Answer from the drawing. Dimensions are ordinates in mm from the lowest x, y and z of the part. Give positions to 0.01 mm unless a question says otherwise; leave off trailing zeros. Loops run counter-clockwise (first coordinate to the right, second up) from the corner with the lowest first, then second, coordinate; pieces in that order, holes last. Notation, with made-up numbers: (38, 86) - (94, 86) arc R24 ccw to (94, 98) - close; hole circle Ø7 at (85.25, 29). An arc over 180 degrees is marked (long way). Put each result on its own line as item: value. Start each with the question number.
1. Consider L1, parallel to X at y = 2.35, z = 25.4; L2, parallel to Z at x = 431.8, y = 1.75; L3, parallel to Z at x = 393.5, y = 20.25 (3 decimals). Determine where each line is inside the solid, lowest interval first. Write a range as from..to.
2. A cutting plane is placed at C-C, the plane z = 8.5. Determine the outline of the cut face in (x, y) (3 decimals).
3. A cutting plane is placed at A-A, the plane y = 17.25. Determine the outline of the cut face in (x, z) (3 decimals).
4. A cutting plane is placed at B-B, the plane x = 71. Determine the outline of the cut face in (y, z) (3 decimals), plus the area to 3 significant figures.
5. For a pull along Z with two mould halves and no side action, classify the marked faces 1, 2, 3 and 4 as released by +Z, released by -Z, zero draft, split by the parting line, or undercut.
6. Given pin 1 Ø8.5 at (x, z) = (25.4, 25.4) entering from +Y (3 decimals); pin 2 Ø2.5 at (y, z) = (14, 50) entering from +X; pin 3 Ø1.6 at (y, z) = (10, 49) entering from -X, each flat-ended and moving along its own axis, determine where each tip first touches the part or whether it passes through.
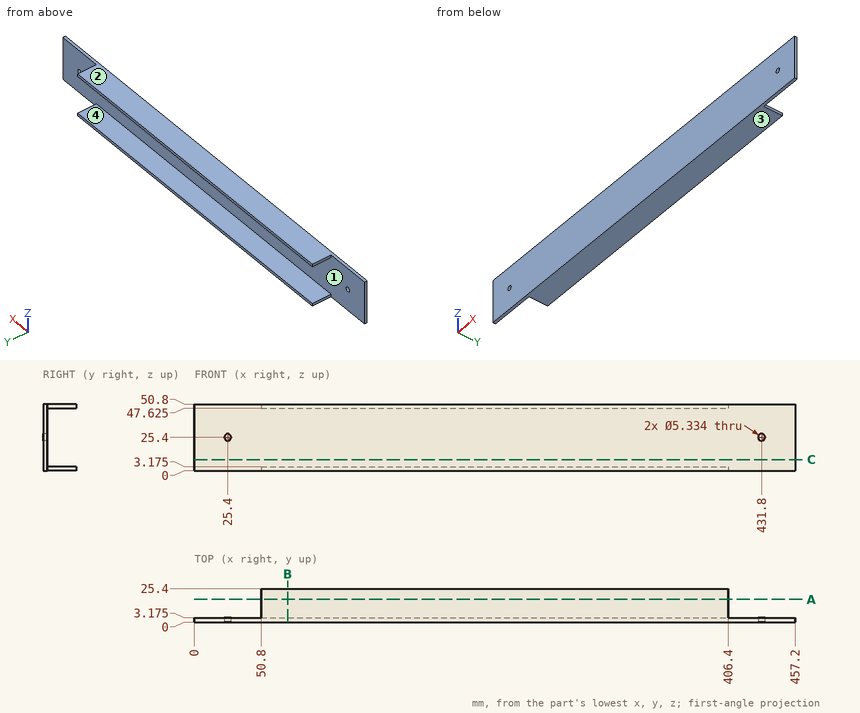
Return value:
1. L1: x = 0..22.73, 28.07..429.13, 434.47..457.2
1. L2: z = 0..22.73, 28.07..50.8
1. L3: z = 0..3.175, 47.625..50.8
2. outline: (0, 0) - (457.2, 0) - (457.2, 3.175) - (0, 3.175) - close
3. outline: (50.8, 0) - (406.4, 0) - (406.4, 3.175) - (50.8, 3.175) - close; (50.8, 47.625) - (406.4, 47.625) - (406.4, 50.8) - (50.8, 50.8) - close
4. outline: (0, 0) - (25.4, 0) - (25.4, 3.175) - (3.175, 3.175) - (3.175, 47.625) - (25.4, 47.625) - (25.4, 50.8) - (0, 50.8) - close
4. area: 302 mm2
5. face 1: undercut
5. face 2: released by +Z
5. face 3: released by -Z
5. face 4: undercut
6. pin 1: stops at y = 3.175
6. pin 2: stops at x = 406.4
6. pin 3: stops at x = 50.8
